Can you work these out from the drawing? Everything is in mm from the part's minimum corner. A direction names the side the tool comes from. Round coordinates to 2 decimals unless told otherwise and drop trailing zeros. Write each loop counter-clockwise with the first axis right and the second up, starting at its lowest first coordinate (ties: lowest second). Pieces come first, ordered by that corner, then holes. Notation, with made-up numbers: M 62,-24 L 79,-24 A17 cw 79,-9 Z; hole C 50.5,58 d1. An arc over 180 degrees is marked long. Answer in a Markdown table with one row per item. Add a question column.
(1) Suppose I cut it at A-A, the plane x = 15. Write out the boundary of the cut face in (y, z), then the cut area to 3 significant figures.
(2) If we mould it in two halves opening along X, with no side actions, what happens to the marked faces 3, 4 and 5? For each: released by +X, released by -X, zero draft, split by the parting line, or undercut.
(3) If I drill on probe 1 along Y at (x, z) = (32, 9.5); probe 2 along Z at (x, y) = (28.5, 15.5), over which ranges is the centre line in solid material (lowest first)?
(4) For the marked faces 1 and 2, which set-ups out of +Z, -Z, +X, -X, +Y, -Y let a thin tool reach every point of the face, with its end or its side?
(5) I'm going to push flat-ended pins straight in: pin 1 (4 mm diameter, centred on x = 8, y = 11.5, fed in from +Z); pin 2 (3 mm diameter, centred on x = 20, z = 8.5, fed in from +Y). Where does each tip first touch, or does it pass through?
(6) Suppose I cut it at B-B, the plane z = 14.5. Write out the boundary of the cut face in (x, y) (3 decimals).
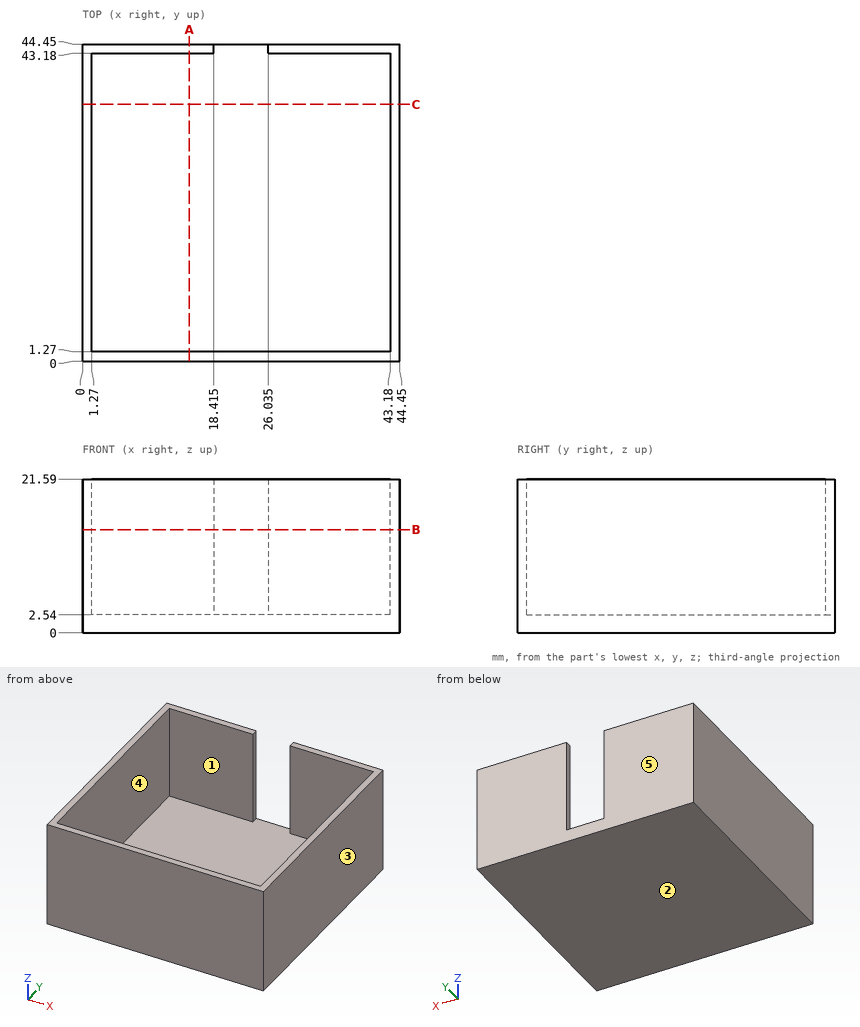
Calculated:
| question | item | result |
|---|---|---|
| 1 | outline | M 0,0 L 44.45,0 L 44.45,21.59 L 43.18,21.59 L 43.18,2.54 L 1.27,2.54 L 1.27,21.59 L 0,21.59 Z |
| 1 | area | 161 mm² |
| 2 | face 3 | released by +X |
| 2 | face 4 | undercut |
| 2 | face 5 | zero draft |
| 3 | probe 1 | 0 to 1.27, 43.18 to 44.45 |
| 3 | probe 2 | 0 to 2.54 |
| 4 | face 1 | +Z |
| 4 | face 2 | -Z, +X, -X, +Y, -Y |
| 5 | pin 1 | z = 2.54 |
| 5 | pin 2 | y = 1.27 |
| 6 | outline | M 0,0 L 44.45,0 L 44.45,44.45 L 26.035,44.45 L 26.035,43.18 L 43.18,43.18 L 43.18,1.27 L 1.27,1.27 L 1.27,43.18 L 18.415,43.18 L 18.415,44.45 L 0,44.45 Z |
